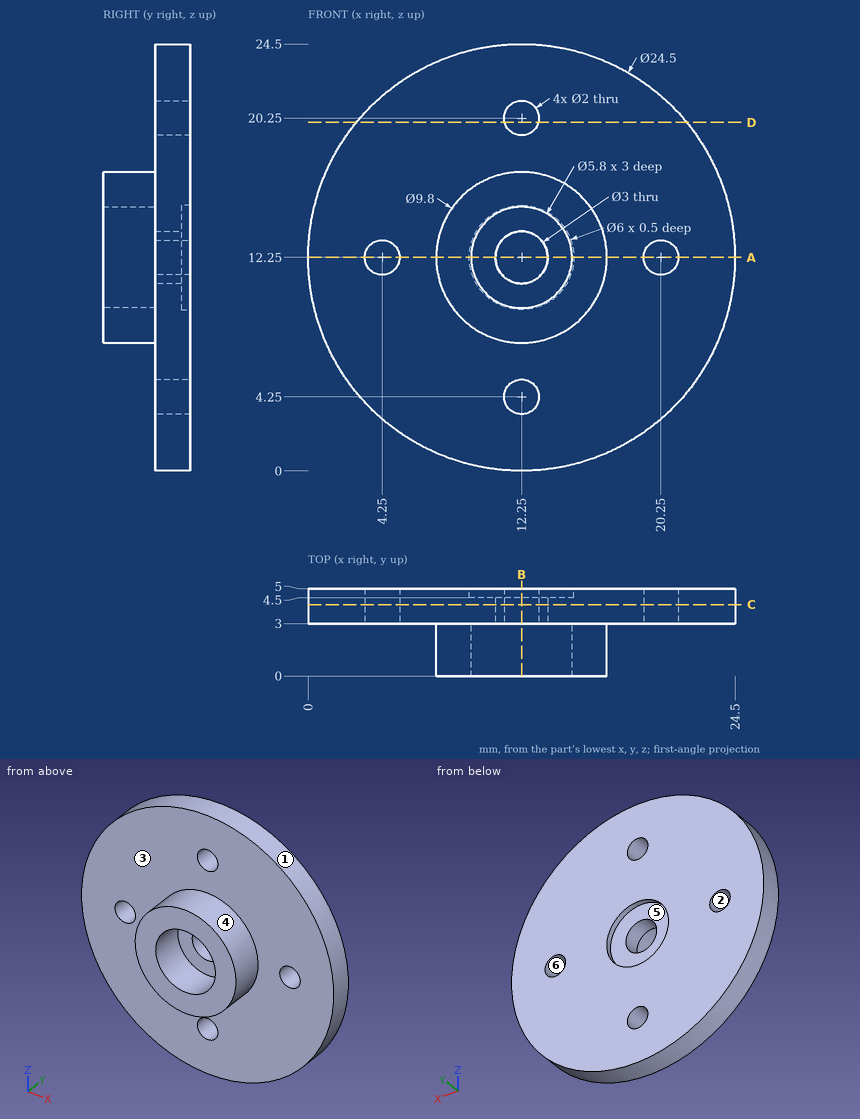
Geometry check sheet. Reference: drawing and pictorial views, mm from the part's lowest x, y, z. A direction names the side the tool comes from. Give positions to 0.01 mm unless a question says otherwise; leave off trailing zeros. Order: outer loops, then holes, each group sorted by start corner. A loop starts at its lowest first (then second) coordinate and runs counter-clockwise, first axis right, second up. Notation, with made-up numbers: M 44.25,-27 L 63.25,-27 A28 cw 63.25,8 Z; hole C -30.5,58 d5. An arc over 180 degrees is marked long. Answer in a Markdown table with one row per item. Add a question column.
Item 1: Section check B-B, the plane x = 12.25. Enter the section's corners in (y, z).
Item 2: Gauge pin test, flat ends, axial feed: pin 1 (2 mm diameter, centred on x = 18.5, y = 3, fed in from +Z); pin 2 (1 mm diameter, centred on x = 7.5, z = 6, fed in from -Y); pin 3 (1.2 mm diameter, centred on x = 20.25, z = 12.25, fed in from +Y); pin 4 (5 mm diameter, centred on x = 12.25, z = 12.25, fed in from +Y). Record the tip position at first contact, or that the pin passes through.
Item 3: Section check D-D, the plane z = 20. Enter the section's corners in (x, y), and give its area (3 significant figures).
Item 4: Section check C-C, the plane y = 4.1. Enter the section's corners in (x, z).
Item 5: Tool access check on the marked faces 4, 5 and 6. Record the directions out of +Z, -Z, +X, -X, +Y, -Y that give a thin tool (end or side, any length) a straight path to the whole face; none if there is none.
Item 6: Mould release check, pull along Z, two halves, no side actions. Record for the marked faces 1, 2 and 3: released by +Z, released by -Z, zero draft, split by the parting line, or undercut.
Item 7: Scan lines: probe 1 along X at (y, z) = (4.1, 12.25); probe 2 along X at (y, z) = (4.75, 12.25); probe 3 along Z at (x, y) = (10, 1.2). Record each from-to range of solid material in increasing order. Write a range as from..to.
Item 8: Section check A-A, the plane z = 12.25. Enter the section's corners in (x, y), and give its area (3 significant figures).
Filled sheet:
| question | item | result |
|---|---|---|
| 1 | outline | M 0,7.35 L 3,7.35 L 3,5.25 L 5,5.25 L 5,9.25 L 4.5,9.25 L 4.5,10.75 L 3,10.75 L 3,9.35 L 0,9.35 Z; M 0,15.15 L 3,15.15 L 3,13.75 L 4.5,13.75 L 4.5,15.25 L 5,15.25 L 5,19.25 L 3,19.25 L 3,17.15 L 0,17.15 Z; M 3,0 L 5,0 L 5,3.25 L 3,3.25 Z; M 3,21.25 L 5,21.25 L 5,24.5 L 3,24.5 Z |
| 2 | pin 1 | stops at z = 23.32 |
| 2 | pin 2 | stops at y = 3 |
| 2 | pin 3 | passes through |
| 2 | pin 4 | stops at y = 4.5 |
| 3 | outline | M 2.76,3 L 11.28,3 L 11.28,5 L 2.76,5 Z; M 13.22,3 L 21.74,3 L 21.74,5 L 13.22,5 Z |
| 3 | area | 34.1 mm^2 |
| 4 | outline | C 12.25,12.25 d24.5; hole C 4.25,12.25 d2; hole C 12.25,12.25 d3; hole C 12.25,4.25 d2; hole C 12.25,20.25 d2; hole C 20.25,12.25 d2 |
| 5 | face 4 | -Y |
| 5 | face 5 | +Y |
| 5 | face 6 | +Y, -Y |
| 6 | face 1 | split by the parting line |
| 6 | face 2 | undercut |
| 6 | face 3 | zero draft |
| 7 | probe 1 | x = 0..3.25, 5.25..10.75, 13.75..19.25, 21.25..24.5 |
| 7 | probe 2 | x = 0..3.25, 5.25..9.25, 15.25..19.25, 21.25..24.5 |
| 7 | probe 3 | z = 7.9..10.42, 14.08..16.6 |
| 8 | outline | M 0,3 L 3.25,3 L 3.25,5 L 0,5 Z; M 5.25,3 L 7.35,3 L 7.35,0 L 9.35,0 L 9.35,3 L 10.75,3 L 10.75,4.5 L 9.25,4.5 L 9.25,5 L 5.25,5 Z; M 13.75,3 L 15.15,3 L 15.15,0 L 17.15,0 L 17.15,3 L 19.25,3 L 19.25,5 L 15.25,5 L 15.25,4.5 L 13.75,4.5 Z; M 21.25,3 L 24.5,3 L 24.5,5 L 21.25,5 Z |
| 8 | area | 45.5 mm^2 |
